```python
from build123d import *

# Parameters (mm, degrees)
F0_W     = 20
F0_H     = 40
F1_DEPTH = 6
F3_D     = 3.3
F3_DEPTH = 10
F3_TIP   = 0.9914200214


with BuildPart() as f1:
    # F0 (on Front) → F1 (new body)
    with BuildSketch(Plane.XZ):
        Rectangle(F0_W, F0_H)
    extrude(amount=F1_DEPTH)

    # F3
    with Locations(Plane.XZ.offset(6)):
        with Locations((-7.5, 15), (7.5, 15), (7.5, -15), (-7.5, -15)):
            Hole(F3_D / 2, depth=F3_DEPTH)
            with Locations((0, 0, -(F3_DEPTH + F3_TIP / 2))):  # 118° drill point
                Cone(0, F3_D / 2, F3_TIP, mode=Mode.SUBTRACT)


solid = f1.part
```
Can you work these out from the model? Positions are in its coordinate system, mm. Round coordinates to 2 decimals unless told otherwise and drop trailing zeros. Loops run counter-clockwise (first coordinate to the right, second up) from the corner with the lowest first, then second, coordinate; pieces in that order, holes last.
Item 1: Suppose I cut it at A-A, the plane y = -5.45. Write out the boundary of the cut face in (x, z).
Item 2: If we mould it in two halves opening along Z, with no side actions, what happens to faces 1 (the flat face through (0, 0, 0)), 2 (the flat face through (0, -3, 20)), 3 (the cylindrical face through (-6.284, -2.958, -13.885))? For each: +Z half, -Z half, draft (parallel to the pull), parting line (faces both ways), or undercut.
Item 3: Suppose I cut it at C-C, the plane z = 15. Write out the boundary of the cut face in (x, y).
Item 4: Suppose I cut it at B-B, the plane x = -7.5. Write out the boundary of the cut face in (y, z), then the cut area to 3 significant figures.
Item 5: Please list where these lines run through material, in increasing order: L1, parallel to Z at x = 7.5, y = -3.65; L2, parallel to Z at x = -8.25, y = -5.15; L3, parallel to X at y = -0.45, z = -15.5.
Reported:
1. outline: (-10, -20) - (10, -20) - (10, 20) - (-10, 20) - close; hole circle Ø3.3 at (-7.5, -15); hole circle Ø3.3 at (-7.5, 15); hole circle Ø3.3 at (7.5, -15); hole circle Ø3.3 at (7.5, 15)
2. face 1: draft
2. face 2: +Z half
2. face 3: undercut
3. outline: (-10, -6) - (-9.15, -6) - (-9.15, 0) - (-10, 0) - close; (-5.85, -6) - (5.85, -6) - (5.85, 0) - (-5.85, 0) - close; (9.15, -6) - (10, -6) - (10, 0) - (9.15, 0) - close
4. outline: (-6, -20) - (0, -20) - (0, -16.65) - (-6, -16.65) - close; (-6, -13.35) - (0, -13.35) - (0, 13.35) - (-6, 13.35) - close; (-6, 16.65) - (0, 16.65) - (0, 20) - (-6, 20) - close
4. area: 200 mm2
5. L1: z = -20 to -16.65, -13.35 to 13.35, 16.65 to 20
5. L2: z = -20 to -16.47, -13.53 to 13.53, 16.47 to 20
5. L3: x = -10 to -9.07, -5.93 to 5.93, 9.07 to 10
